Source: CAD feature listing. Evaluate the final solid. Frame: model axes, mm. Face numbers are marked on the shaded views. Give positions to 0.01 mm unless a question says otherwise; leave off trailing zeros. Write each loop counter-clockwise with the first axis right and the second up, starting at its lowest first coordinate (ties: lowest second). Pieces come first, ordered by that corner, then holes. Notation, with made-up numbers: (2, 20) -> (58, 20) arc R14 cw to (58, 38) -> close; hole circle Ø9 at (58, -17). An arc over 180 degrees is marked (long way). Use a Markdown table: item, result. Add a question column.
```python
from build123d import *

# Parameters (mm, degrees)
BASE_CROQUIS_W               = 120
BASE_CROQUIS_H               = 120
BASE_SALIENTE_DEPTH          = 5
ENCAJE_RUEDAS_CROQUIS_W      = 31
ENCAJE_RUEDAS_CROQUIS_H      = 60
ENCAJE_RUEDAS_CORTAR_DEPTH   = 5
CAJA_PLACAS_CROQUIS_1_W      = 58
CAJA_PLACAS_CROQUIS_1_H      = 42
CAJA_PLACAS_CROQUIS_1_W_2    = 42
CAJA_PLACAS_CROQUIS_1_H_2    = 32
CAJA_PLACAS_SALIENTE_1_DEPTH = 5
CAJA_PLACAS_CROQUIS_2_W      = 42
CAJA_PLACAS_CROQUIS_2_H      = 32
CAJA_PLACAS_CORTAR_2_DEPTH   = 2.5
CAJA_PLACAS_CROQUIS_3_W      = 58
CAJA_PLACAS_CROQUIS_3_H      = 42
CAJA_PLACAS_SALIENTE_3_DEPTH = 2.5
CAJA_PLACAS_CORTAR_4_DEPTH   = 7.5


with BuildPart() as part:
    # Base-Croquis → Base-Saliente (new body)
    with BuildSketch(Plane(origin=(0, 0, 0), x_dir=(1, 0, 0), z_dir=(0, 1, 0))):
        Rectangle(BASE_CROQUIS_W, BASE_CROQUIS_H)
    extrude(amount=BASE_SALIENTE_DEPTH)

    # Encaje-Ruedas-Croquis → Encaje-Ruedas-Cortar (cut)
    with BuildSketch(Plane(origin=(0, 5, 0), x_dir=(1, 0, 0), z_dir=(0, 1, 0))):
        with Locations((44.5, 30)):
            Rectangle(ENCAJE_RUEDAS_CROQUIS_W, ENCAJE_RUEDAS_CROQUIS_H)
        with Locations((-44.5, 30)):
            Rectangle(ENCAJE_RUEDAS_CROQUIS_W, ENCAJE_RUEDAS_CROQUIS_H)
    extrude(amount=-ENCAJE_RUEDAS_CORTAR_DEPTH, mode=Mode.SUBTRACT)

    # Caja-Placas-Croquis-1 → Caja-Placas-Saliente-1 (add)
    with BuildSketch(Plane(origin=(0, 5, 0), x_dir=(1, 0, 0), z_dir=(0, 1, 0))):
        with Locations((0, 24)):
            Rectangle(CAJA_PLACAS_CROQUIS_1_W, CAJA_PLACAS_CROQUIS_1_H)
        with Locations((0, 24)):
            Rectangle(CAJA_PLACAS_CROQUIS_1_W_2, CAJA_PLACAS_CROQUIS_1_H_2, mode=Mode.SUBTRACT)
    extrude(amount=CAJA_PLACAS_SALIENTE_1_DEPTH)

    # Caja-Placas-Croquis-2 → Caja-Placas-Cortar-2 (cut)
    with BuildSketch(Plane(origin=(0, 5, 0), x_dir=(1, 0, 0), z_dir=(0, 1, 0))):
        with Locations((0, 24)):
            Rectangle(CAJA_PLACAS_CROQUIS_2_W, CAJA_PLACAS_CROQUIS_2_H)
    extrude(amount=-CAJA_PLACAS_CORTAR_2_DEPTH, mode=Mode.SUBTRACT)

    # Caja-Placas-Croquis-3 → Caja-Placas-Saliente-3 (add)
    with BuildSketch(Plane(origin=(0, 10, 0), x_dir=(1, 0, 0), z_dir=(0, 1, 0))):
        with Locations((0, 24)):
            Rectangle(CAJA_PLACAS_CROQUIS_3_W, CAJA_PLACAS_CROQUIS_3_H)
    extrude(amount=CAJA_PLACAS_SALIENTE_3_DEPTH)

    # Caja-Placas-Croquis-4 → Caja-Placas-Cortar-4 (cut)
    with BuildSketch(Plane(origin=(0, 12.5, 0), x_dir=(1, 0, 0), z_dir=(0, 1, 0))):
        Polygon((23.5, 42.5), (26, 42.5), (27.25, 42.5), (27.25, 43.75), (26, 43.75), (26, 45), (-26, 45), (-26, 43.75), (-27.25, 43.75), (-27.25, 42.5), (-26, 42.5), (-23.5, 42.5), (-23.5, 41.25), (-24.75, 41.25), (-24.75, 40), (-23.5, 40), (23.5, 40), (24.75, 40), (24.75, 41.25), (23.5, 41.25), align=None)
    extrude(amount=-CAJA_PLACAS_CORTAR_4_DEPTH, mode=Mode.SUBTRACT)


solid = part.part
```
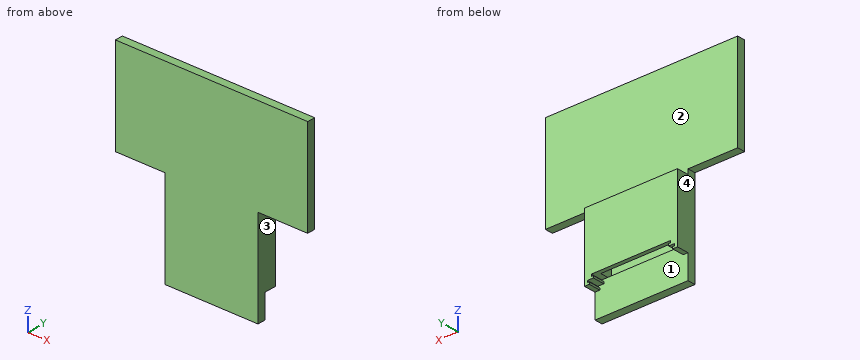
(1) Cut plane B-B on y = 8.5. Return the cut outline in (x, z).
(2) Cut plane D-D on z = -47. Return the cut outline in (x, y).
(3) Material intervals for L1, parallel to Z at x = 35.5, y = 3; L2, parallel to Z at x = -16, y = 7; L3, parallel to Y at x = 14.5, z = -35, sorted ascending.
(4) First-contact query: pin 1 Ø1.4 at (y, z) = (8, -44) entering from -X; pin 2 Ø1 at (x, y) = (-26.5, 7) entering from +Z; pin 3 Ø1 at (y, z) = (7, -44) entering from +X. Flat tips, straight axial feed; report the tip coordinate or a pass-through.
(5) Cut plane A-A on z = -9.5. Return the cut outline in (x, y), then the cut area to 3 significant figures.
(6) Mould query, pull axis X, two halves, no side actions, for the marked faces 1, 2, 3 and 4. Classes: +X half, -X half, draft (parallel to the pull), parting line (faces both ways), or undercut.
(7) Cut plane C-C on x = -12. Return the cut outline in (y, z), then the cut area to 4 significant figures.
Output:
| question | item | result |
|---|---|---|
| 1 | outline | (-29, -45) -> (-26, -45) -> (-26, -43.75) -> (-27.25, -43.75) -> (-27.25, -42.5) -> (-23.5, -42.5) -> (-23.5, -41.25) -> (-24.75, -41.25) -> (-24.75, -40) -> (-21, -40) -> (-21, -8) -> (21, -8) -> (21, -40) -> (24.75, -40) -> (24.75, -41.25) -> (23.5, -41.25) -> (23.5, -42.5) -> (27.25, -42.5) -> (27.25, -43.75) -> (26, -43.75) -> (26, -45) -> (29, -45) -> (29, -3) -> (-29, -3) -> close |
| 2 | outline | (-29, 0) -> (29, 0) -> (29, 5) -> (-29, 5) -> close |
| 3 | L1 | 0 to 60 |
| 3 | L2 | -8 to -3 |
| 3 | L3 | 0 to 2.5, 10 to 12.5 |
| 4 | pin 1 | x = -29 |
| 4 | pin 2 | z = -3 |
| 4 | pin 3 | x = 29 |
| 5 | outline | (-29, 0) -> (29, 0) -> (29, 12.5) -> (-29, 12.5) -> close; hole (-21, 2.5) -> (21, 2.5) -> (21, 10) -> (-21, 10) -> close |
| 5 | area | 410 mm^2 |
| 6 | face 1 | undercut |
| 6 | face 2 | draft |
| 6 | face 3 | +X half |
| 6 | face 4 | -X half |
| 7 | outline | (0, -60) -> (5, -60) -> (5, -40) -> (2.5, -40) -> (2.5, -8) -> (10, -8) -> (10, -40) -> (12.5, -40) -> (12.5, -3) -> (5, -3) -> (5, 60) -> (0, 60) -> close |
| 7 | area | 637.5 mm^2 |
